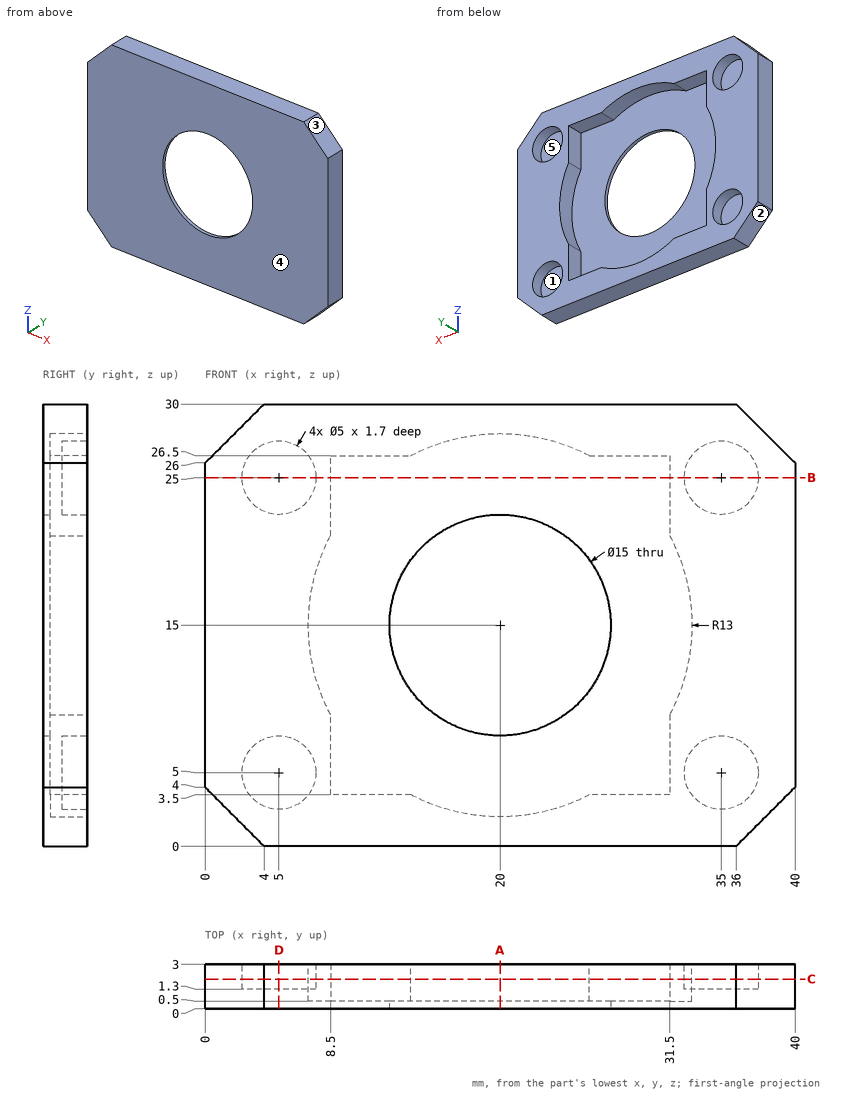
Input: dimensioned drawing with shaded views. Units: mm. Origin: part minimum x, y, z. A direction names the side the tool comes from. Coordinates: 2 decimals unless noted, no trailing zeros. Order: outer loops, then holes, each group sorted by start corner. A loop starts at its lowest first (then second) coordinate and runs counter-clockwise, first axis right, second up. Notation, with made-up numbers: (22.5, 65) -> (58.5, 65) arc R29 ccw to (58.5, 92) -> close; hole circle Ø9 at (35.25, -14). An arc over 180 degrees is marked (long way). Answer in a Markdown table with one row per item.
Item 1: Section A-A on x = 20. Output: boundary loops of the cut face in (y, z).
Return value:
| item | result |
|---|---|
| outline | (0, 0) -> (3, 0) -> (3, 2) -> (0.5, 2) -> (0.5, 7.5) -> (0, 7.5) -> close; (0, 22.5) -> (0.5, 22.5) -> (0.5, 28) -> (3, 28) -> (3, 30) -> (0, 30) -> close |
Item 2: Ray query, L1, parallel to X at y = 2, z = 5; L2, parallel to Z at x = 35, y = 2.25; L3, parallel to Z at x = 12.5, y = 1.3. Return the intervals inside material, ascending.
Return value:
| item | result |
|---|---|
| L1 | x = 0 to 2.5, 7.5 to 8.5, 31.5 to 32.5, 37.5 to 40 |
| L2 | z = 0 to 2.5, 7.5 to 22.5, 27.5 to 30 |
| L3 | z = 0 to 3.5, 26.5 to 30 |
Item 3: Contact query for a flat-ended pin moving along its axis: P1, Ø2.5, axis at x = 34, z = 25.5, coming from the +Y side. Output: stop coordinate, or through.
Return value:
| item | result |
|---|---|
| P1 | stops at y = 1.3 |
Item 4: Draft query along Z for the marked faces 3, 4 and 5. Return one class per face: released by +Z, released by -Z, zero draft, split by the parting line, or undercut.
Return value:
| item | result |
|---|---|
| face 3 | released by +Z |
| face 4 | zero draft |
| face 5 | undercut |
Item 5: Section C-C on y = 2. Output: boundary loops of the cut face in (x, z), plus the area to 3 significant figures.
Return value:
| item | result |
|---|---|
| outline | (0, 4) -> (4, 0) -> (36, 0) -> (40, 4) -> (40, 26) -> (36, 30) -> (4, 30) -> (0, 26) -> close; hole circle Ø5 at (5, 5); hole circle Ø5 at (5, 25); hole (8.5, 3.5) -> (13.94, 3.5) arc R13 ccw to (26.06, 3.5) -> (31.5, 3.5) -> (31.5, 8.94) arc R13 ccw to (31.5, 21.06) -> (31.5, 26.5) -> (26.06, 26.5) arc R13 ccw to (13.94, 26.5) -> (8.5, 26.5) -> (8.5, 21.06) arc R13 ccw to (8.5, 8.94) -> close; hole circle Ø5 at (35, 5); hole circle Ø5 at (35, 25) |
| area | 511 mm² |
Item 6: Access query for the marked faces 1 and 2. Directions: +Z, -Z, +X, -X, +Y, -Y. A direction counts if a zero-diameter tool reaches every point of the face in a straight line with its end or side. Return the directions, or none.
Return value:
| item | result |
|---|---|
| face 1 | +Y |
| face 2 | -Z, -X, +Y, -Y |
Item 7: Section B-B on z = 25. Output: boundary loops of the cut face in (x, y).
Return value:
| item | result |
|---|---|
| outline | (0, 0) -> (40, 0) -> (40, 3) -> (37.5, 3) -> (37.5, 1.3) -> (32.5, 1.3) -> (32.5, 3) -> (31.5, 3) -> (31.5, 0.5) -> (8.5, 0.5) -> (8.5, 3) -> (7.5, 3) -> (7.5, 1.3) -> (2.5, 1.3) -> (2.5, 3) -> (0, 3) -> close |
Item 8: Section D-D on x = 5. Output: boundary loops of the cut face in (y, z), plus the area to 3 significant figures.
Return value:
| item | result |
|---|---|
| outline | (0, 0) -> (3, 0) -> (3, 2.5) -> (1.3, 2.5) -> (1.3, 7.5) -> (3, 7.5) -> (3, 22.5) -> (1.3, 22.5) -> (1.3, 27.5) -> (3, 27.5) -> (3, 30) -> (0, 30) -> close |
| area | 73.0 mm² |
